Part model, mm, in its own coordinate system. A direction names the side the tool comes from. Give positions to 0.01 mm unless a question says otherwise; leave off trailing zeros. Write each loop counter-clockwise with the first axis right and the second up, starting at its lowest first coordinate (ties: lowest second). Pieces come first, ordered by that corner, then holes. Notation, with made-up numbers: (-33.5, 52.5) - (-23.5, 52.5) arc R8 cw to (-23.5, 66.5) - close; hole circle Ø7 at (-30, 72). An arc over 180 degrees is marked (long way). Answer in a Markdown table with one row per item. Add a question column.
1. Drop flat-ended pins along their axis: pin 1 Ø1.5 at (x, y) = (1, 97) entering from +Z; pin 2 Ø1.5 at (x, z) = (2, 51) entering from +Y; pin 3 Ø4 at (y, z) = (5, 219.13) entering from +X; pin 4 Ø1 at (x, y) = (1.5, -100) entering from -Z. Give the stop position or say it passes through.
2. Band-saw the part on B-B on x = 0.9. State how many separate pieces and enclosed holes the cut face has, plus the area to 3 significant figures.
3. Pull direction Y, two halves, no side cores. Call faces 3 (the flat face through (1.6, -13.3, 210.7)), 4 (the flat face through (3.18, -90, 109)), 5 (the flat face through (1.57, 12.99, 211.49)), 6 (the flat face through (1.57, 64.51, 136.13)): released by +Y, released by -Y, zero draft, split by the parting line, or undercut.
4. Band-saw the part on C-C on z = 70.5. Write the cut outline in (x, y).
5. Band-saw the part on A-A on y = -260. Write the cut outline in (x, z).
6. Probe line 1 along Z through (x, y) = (2, 5); line 2 along Z through (x, y) = (0.75, 0); line 3 along Y through (x, z) = (0.2, 16). List the from-to ranges inside material, lowest first.
7. Which spindle directions (+Z, -Z, +X, -X, +Y, -Y) get a long thin tool onto all of the face, cutting with end or side? Do faces 1 (the flat face through (1.568, 81.145, 161.18)), 2 (the flat face through (1.568, 68.782, 146.663)). Say none if no direction does.
```python
from build123d import *

# Parameters (mm, degrees)
SKETCH3_R                           = 4.765
SKETCH3_R_2                         = 1.25
SKETCH3_R_3                         = 18.5
BOSS_ROCKER_BASE_DEPTH              = 3.18
SKETCH4_R                           = 1.25
CUT_MOTOR_HOLES_SHAFT_SUPPORT_DEPTH = 3.18
SKETCH5_R                           = 1.25
CUT_SUPPORT_HOLES_DEPTH             = 3.18
CUT_LIGHTENING_HOLES_DEPTH          = 3.18


with BuildPart() as part:
    # Sketch3 → Boss-rocker base (new body)
    with BuildSketch(Plane.YZ):
        with BuildLine():
            Line((-19.740098585, 194.326279503), (-247.886058825, 27.445444598))
            ThreePointArc((-247.886058825, 27.445444598), (-284.213703097, -17.711481653), (-230.174577172, 3.231741502))
            Line((-230.174577172, 3.231741502), (-1.602441241, 170.424309102))
            ThreePointArc((-1.602441241, 170.424309102), (1.066332673, 171.380668673), (3.826130086, 170.732211983))
            Line((3.826130086, 170.732211983), (126.91354691, 100.548260636))
            ThreePointArc((126.91354691, 100.548260636), (130.710275653, 100.069186741), (133.733724692, 102.415122982))
            Line((133.733724692, 102.415122982), (143.640355564, 119.789203239))
            ThreePointArc((143.640355564, 119.789203239), (144.119429459, 123.585931982), (141.773493218, 126.609381021))
            Line((141.773493218, 126.609381021), (18.794188293, 196.731687397))
            Line((18.794188293, 196.731687397), (7.025536002, 226.658847865))
            ThreePointArc((7.025536002, 226.658847865), (5.922779586, 228.040238472), (4.233648495, 228.560957093))
            Line((4.233648495, 228.560957093), (-4.233648495, 228.560957093))
            ThreePointArc((-4.233648495, 228.560957093), (-5.922779586, 228.040238472), (-7.025536002, 226.658847865))
            Line((-7.025536002, 226.658847865), (-19.740098585, 194.326279503))
        make_face()
        with Locations((0, 190.180957093)):
            Circle(SKETCH3_R, mode=Mode.SUBTRACT)
        with Locations((130, 116.055478547)):
            Circle(SKETCH3_R, mode=Mode.SUBTRACT)
        with Locations((-5, 219.130957093)):
            Circle(SKETCH3_R_2, mode=Mode.SUBTRACT)
        with Locations((5, 219.130957093)):
            Circle(SKETCH3_R_2, mode=Mode.SUBTRACT)
        with Locations((-260, 0)):
            Circle(SKETCH3_R_3, mode=Mode.SUBTRACT)
    extrude(amount=BOSS_ROCKER_BASE_DEPTH)

    # Sketch4 → Cut-motor holes + shaft support (cut)
    with BuildSketch(Plane.YZ):
        with Locations((0, 180.656752709)):
            Circle(SKETCH4_R)
        with Locations((-8.24, 194.928851363)):
            Circle(SKETCH4_R)
        with Locations((8.24, 194.928851363)):
            Circle(SKETCH4_R)
    extrude(amount=CUT_MOTOR_HOLES_SHAFT_SUPPORT_DEPTH, mode=Mode.SUBTRACT)

    # Sketch5 → Cut-support holes (cut)
    with BuildSketch(Plane.YZ):
        with Locations((-173.097100025, 78.211048963)):
            Circle(SKETCH5_R)
        with Locations((-159.140452483, 59.130650922)):
            Circle(SKETCH5_R)
        with Locations((-94.167013372, 106.656461829)):
            Circle(SKETCH5_R)
        with Locations((-108.123660914, 125.73685987)):
            Circle(SKETCH5_R)
        with Locations((-221.524503751, 42.788087462)):
            Circle(SKETCH5_R)
        with Locations((-207.567856209, 23.707689422)):
            Circle(SKETCH5_R)
        with Locations((-45.739607178, 142.079425135)):
            Circle(SKETCH5_R)
        with Locations((-59.69625472, 161.159823175)):
            Circle(SKETCH5_R)
        with Locations((103.007538851, 117.839995969)):
            Circle(SKETCH5_R)
        with Locations((114.717176541, 138.376158833)):
            Circle(SKETCH5_R)
        with Locations((62.594935771, 168.096051448)):
            Circle(SKETCH5_R)
        with Locations((50.885298081, 147.559888585)):
            Circle(SKETCH5_R)
        with Locations((-280.985209351, -15.349950766)):
            Circle(SKETCH5_R)
    extrude(amount=CUT_SUPPORT_HOLES_DEPTH, mode=Mode.SUBTRACT)

    # Sketch6 → Cut-lightening holes (cut)
    with BuildSketch(Plane.YZ):
        with BuildLine():
            Line((-79.983471427, 142.368791683), (-61.979782767, 147.316428458))
            ThreePointArc((-61.979782767, 147.316428458), (-59.811067724, 146.534457497), (-59.819745898, 144.229088067))
            Line((-59.819745898, 144.229088067), (-67.122963599, 133.95613022))
            ThreePointArc((-67.122963599, 133.95613022), (-67.760393878, 133.378682327), (-68.581402, 133.122344477))
            Line((-68.581402, 133.122344477), (-77.604831251, 132.34516891))
            ThreePointArc((-77.604831251, 132.34516891), (-78.919471752, 132.69660063), (-79.704956379, 133.807815192))
            Line((-79.704956379, 133.807815192), (-81.381998087, 139.910311831))
            ThreePointArc((-81.381998087, 139.910311831), (-81.191902606, 141.429196112), (-79.983471427, 142.368791683))
        make_face()
        with BuildLine():
            Line((-23.474916203, 177.031971532), (-31.234891161, 177.031971532))
            ThreePointArc((-31.234891161, 177.031971532), (-32.91387852, 176.518133523), (-34.017714198, 175.152639164))
            Line((-34.017714198, 175.152639164), (-37.880265406, 165.561216901))
            ThreePointArc((-37.880265406, 165.561216901), (-37.857627092, 163.26522791), (-36.218110002, 161.657726231))
            Line((-36.218110002, 161.657726231), (-33.122502329, 160.411097438))
            ThreePointArc((-33.122502329, 160.411097438), (-31.392547815, 160.256443753), (-29.866816812, 161.086386695))
            Line((-29.866816812, 161.086386695), (-20.893300564, 170.176925526))
            ThreePointArc((-20.893300564, 170.176925526), (-20.132536099, 171.500594144), (-20.121734598, 173.027271748))
            Line((-20.121734598, 173.027271748), (-20.568332353, 174.774783973))
            ThreePointArc((-20.568332353, 174.774783973), (-21.634866927, 176.401405781), (-23.474916203, 177.031971532))
        make_face()
        with BuildLine():
            Line((-123.842513182, 102.258163939), (-127.383477271, 102.258163939))
            ThreePointArc((-127.383477271, 102.258163939), (-128.217930269, 102.139776022), (-128.986523832, 101.793956069))
            Line((-128.986523832, 101.793956069), (-137.87452461, 96.175246667))
            ThreePointArc((-137.87452461, 96.175246667), (-138.681600876, 95.425877769), (-139.163866001, 94.435753436))
            Line((-139.163866001, 94.435753436), (-140.452603638, 89.754685534))
            ThreePointArc((-140.452603638, 89.754685534), (-140.168511172, 87.476227852), (-138.356514585, 86.065998684))
            Line((-138.356514585, 86.065998684), (-135.427175254, 85.259526758))
            ThreePointArc((-135.427175254, 85.259526758), (-134.189854142, 85.184508534), (-133.027829794, 85.61612258))
            Line((-133.027829794, 85.61612258), (-123.19292846, 91.833432183))
            ThreePointArc((-123.19292846, 91.833432183), (-122.319685125, 92.675710701), (-121.851449189, 93.794970338))
            Line((-121.851449189, 93.794970338), (-120.89798735, 98.683909964))
            ThreePointArc((-120.89798735, 98.683909964), (-121.527047578, 101.165680397), (-123.842513182, 102.258163939))
        make_face()
        with BuildLine():
            Line((-173.179518759, 50.529751316), (-187.062617136, 41.348992712))
            ThreePointArc((-187.062617136, 41.348992712), (-188.206182034, 41.377149334), (-188.575130176, 42.459928509))
            Line((-188.575130176, 42.459928509), (-186.300929891, 50.354284082))
            ThreePointArc((-186.300929891, 50.354284082), (-184.055505641, 53.265590831), (-180.426317386, 53.854343461))
            Line((-180.426317386, 53.854343461), (-173.517109299, 52.340698989))
            ThreePointArc((-173.517109299, 52.340698989), (-172.74804587, 51.547125046), (-173.179518759, 50.529751316))
        make_face()
        with BuildLine():
            Line((-227.536912906, 31.443521835), (-233.642526561, 26.214778226))
            ThreePointArc((-233.642526561, 26.214778226), (-234.07149562, 25.699434586), (-234.306028267, 25.071272219))
            Line((-234.306028267, 25.071272219), (-235.520501126, 18.719097413))
            ThreePointArc((-235.520501126, 18.719097413), (-235.489047738, 17.830056904), (-235.075165658, 17.0426028))
            Line((-235.075165658, 17.0426028), (-234.178175321, 15.995185513))
            ThreePointArc((-234.178175321, 15.995185513), (-233.016054277, 15.328216057), (-231.693713026, 15.544519522))
            Line((-231.693713026, 15.544519522), (-227.597149989, 17.802325732))
            ThreePointArc((-227.597149989, 17.802325732), (-227.423433386, 17.909992398), (-227.261611665, 18.034825485))
            Line((-227.261611665, 18.034825485), (-219.133655325, 24.995468947))
            ThreePointArc((-219.133655325, 24.995468947), (-218.552793599, 25.837124808), (-218.463915883, 26.855891554))
            ThreePointArc((-218.463915883, 26.855891554), (-221.531743706, 31.287956059), (-226.896432107, 31.812247659))
            ThreePointArc((-226.896432107, 31.812247659), (-227.233851743, 31.657725269), (-227.536912906, 31.443521835))
        make_face()
        with BuildLine():
            Line((85.568117513, 143.181930885), (86.544369033, 149.434919538))
            ThreePointArc((86.544369033, 149.434919538), (86.183746182, 150.922567652), (84.87682125, 151.719494858))
            Line((84.87682125, 151.719494858), (66.429148509, 154.599648582))
            ThreePointArc((66.429148509, 154.599648582), (64.362763101, 153.577467158), (64.632063287, 151.28786437))
            Line((64.632063287, 151.28786437), (73.050048081, 141.906596667))
            ThreePointArc((73.050048081, 141.906596667), (73.74868466, 141.404929088), (74.593412473, 141.243070035))
            Line((74.593412473, 141.243070035), (83.646848899, 141.491195361))
            ThreePointArc((83.646848899, 141.491195361), (84.913320183, 141.989025039), (85.568117513, 143.181930885))
        make_face()
        with BuildLine():
            Line((21.93232317, 175.41253387), (22.178458249, 177.199337176))
            ThreePointArc((22.178458249, 177.199337176), (23.054223795, 178.936124213), (24.811171332, 179.770707856))
            Line((24.811171332, 179.770707856), (32.521378103, 180.648160365))
            ThreePointArc((32.521378103, 180.648160365), (34.247699157, 180.327467884), (35.498857547, 179.095546323))
            Line((35.498857547, 179.095546323), (40.421178328, 170.0023928))
            ThreePointArc((40.421178328, 170.0023928), (40.658302188, 167.718569205), (39.211066927, 165.935990164))
            Line((39.211066927, 165.935990164), (36.27627425, 164.347323378))
            ThreePointArc((36.27627425, 164.347323378), (34.574902041, 163.998048434), (32.965111147, 164.650147857))
            Line((32.965111147, 164.650147857), (23.021241192, 172.667712351))
            ThreePointArc((23.021241192, 172.667712351), (22.115683157, 173.896868902), (21.93232317, 175.41253387))
        make_face()
        with BuildLine():
            Line((1.921390016, 215.785081873), (-1.921390016, 215.785081873))
            ThreePointArc((-1.921390016, 215.785081873), (-2.199739759, 215.700438853), (-2.38384805, 215.475167556))
            Line((-2.38384805, 215.475167556), (-8.248888496, 201.206154542))
            ThreePointArc((-8.248888496, 201.206154542), (-8.149028051, 200.671797182), (-7.620562901, 200.544382574))
            Line((-7.620562901, 200.544382574), (-0.165867561, 203.165811621))
            ThreePointArc((-0.165867561, 203.165811621), (0, 203.194125335), (0.165867561, 203.165811621))
            Line((0.165867561, 203.165811621), (7.620562901, 200.544382574))
            ThreePointArc((7.620562901, 200.544382574), (8.149028051, 200.671797182), (8.248888496, 201.206154542))
            Line((8.248888496, 201.206154542), (2.38384805, 215.475167556))
            ThreePointArc((2.38384805, 215.475167556), (2.199739759, 215.700438853), (1.921390016, 215.785081873))
        make_face()
    extrude(amount=CUT_LIGHTENING_HOLES_DEPTH, mode=Mode.SUBTRACT)


solid = part.part
```
Values:
| question | item | result |
|---|---|---|
| 1 | pin 1 | stops at z = 152.57 |
| 1 | pin 2 | stops at y = -163.84 |
| 1 | pin 3 | stops at x = 3.18 |
| 1 | pin 4 | stops at z = 98.08 |
| 2 | separate pieces | 1 |
| 2 | enclosed holes | 29 |
| 2 | area | 14,200 mm² |
| 3 | face 3 | released by -Y |
| 3 | face 4 | zero draft |
| 3 | face 5 | released by +Y |
| 3 | face 6 | undercut |
| 4 | outline | (0, -189.03) - (3.18, -189.03) - (3.18, -138.21) - (0, -138.21) - close |
| 5 | outline | (0, -30) - (3.18, -30) - (3.18, -18.5) - (0, -18.5) - close; (0, 18.5) - (3.18, 18.5) - (3.18, 30) - (0, 30) - close |
| 6 | line 1 | z = 170.06 to 201.47, 209.11 to 217.88, 220.38 to 228.46 |
| 6 | line 2 | z = 171.2 to 179.41, 181.91 to 185.42, 194.95 to 203.19, 215.79 to 228.56 |
| 6 | line 3 | y = -285.38 to -269.29, -250.71 to -234.18, -230.87 to -212.72 |
| 7 | face 1 | +Z, +X, -X, +Y |
| 7 | face 2 | +X, -X |
